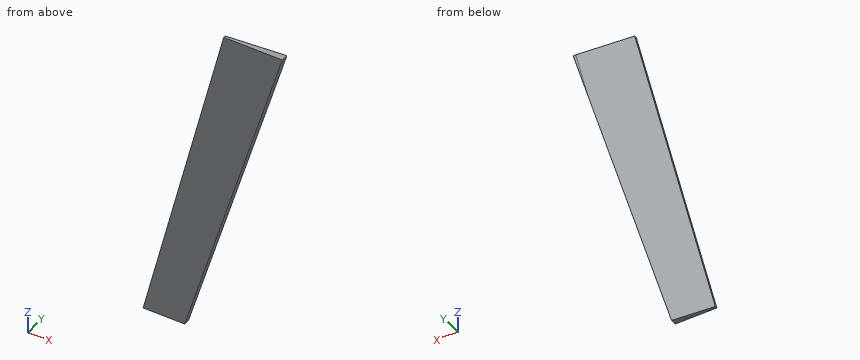
from build123d import *

# Parameters (mm, degrees)
BOSS_EXTRUDE1_DEPTH = 3.81
CHAMFER1_SIZE       = 2.54
CHAMFER1_SIZE2      = 29.032332849


with BuildPart() as part:
    # Sketch2 → Boss-Extrude1 (new body)
    with BuildSketch(Plane(origin=(0, 0, 0), x_dir=(1, 0, 0), z_dir=(0, 1, 0))):
        Polygon((126.581568969, -16.678776649), (178.902552059, -186.601969437), (147.550785663, -186.601969437), (104.349973937, -16.678776649), align=None)
    extrude(amount=BOSS_EXTRUDE1_DEPTH)

    # Chamfer1
    chamfer1_edges = [part.edges().sort_by_distance(p)[0] for p in [
        (125.9503798, 3.81, 101.640373043),
    ]]
    chamfer1_side = [part.faces().sort_by_distance(p)[0] for p in [
        (125.9503798, 1.905, 101.640373043),
    ]]
    chamfer(chamfer1_edges, length=CHAMFER1_SIZE, length2=CHAMFER1_SIZE2, reference=chamfer1_side[0])


solid = part.part
For this review, take the finished solid that the model builds, in its own axes (mm). Round coordinates to 2 decimals unless told otherwise and drop trailing zeros. Order: outer loops, then holes, each group sorted by start corner. A loop starts at its lowest first (then second) coordinate and runs counter-clockwise, first axis right, second up. Notation, with made-up numbers: (74.25, -18) -> (92.25, -18) arc R21 cw to (92.25, 0) -> close; hole circle Ø1 at (50, -1). An arc over 180 degrees is marked (long way). Put each result on its own line as item: value.
Q1. Add section A-A on z = 173. Write out the cut boundary in (x, y), plus the area to 3 significant figures.
Check result:
outline: (144.09, 0) -> (174.71, 0) -> (174.71, 3.81) -> (174.05, 3.81) -> (144.09, 1.27) -> close
area: 78.6 mm2
Q2. Add section B-B on x = 141.5. Write out the cut boundary in (y, z), plus the area to 3 significant figures.
Check result:
outline: (0, 65.13) -> (3.38, 65.13) -> (1.27, 162.8) -> (0, 162.8) -> close
area: 227 mm2
Q3. Add section C-C on y = 2. Write out the cut boundary in (x, z).
Check result:
outline: (112.96, 16.68) -> (126.58, 16.68) -> (178.9, 186.6) -> (156.16, 186.6) -> close
Q4. For probe 1 along Y at (x, z) = (157, 136); probe 2 along Y at (x, z) = (155, 176); probe 3 along X at (y, z) = (0.8, 122.5), list the stretches that pass through material, from the lowest coordinate up. Write a range as [from, to].
Check result:
probe 1: [0, 3.16]
probe 2: [0, 2.13]
probe 3: [131.25, 159.16]
